Verification items for the finished model (mm, model axes). Face numbers are marked on the shaded views. A direction names the side the tool comes from. Give positions to 0.01 mm unless a question says otherwise; leave off trailing zeros. Loops run counter-clockwise (first coordinate to the right, second up) from the corner with the lowest first, then second, coordinate; pieces in that order, holes last. Notation, with made-up numbers: (-17, 9) - (1, 9) arc R8 ccw to (1, 14) - close; hole circle Ø9 at (6.5, 11). An arc over 180 degrees is marked (long way). One line per question, with ' | ' between items. Start each with the question number.
1. Tool access check on the marked faces 4, 5 and 6. Record the directions out of +Z, -Z, +X, -X, +Y, -Y that give a thin tool (end or side, any length) a straight path to the whole face; none if there is none.
2. Depth check by flat-ended pin: pin 1 Ø3 at (y, z) = (17.5, 1) entering from +X; pin 2 Ø1.5 at (y, z) = (29.5, 3.5) entering from -X; pin 3 Ø3 at (y, z) = (43, 4.5) entering from -X; pin 4 Ø3 at (y, z) = (24.5, 2) entering from +X. Enter the tip coordinate at first touch or a pass-through.
3. Section check B-B, the plane y = 9. Enter the section's corners in (x, z), then the cut area to 3 significant figures.
4. Thickness scan on line 1 along Y through (x, z) = (9.35, 3); line 2 along Z through (x, y) = (66.2, 25); line 3 along Y through (x, z) = (70, 0.75). Record the ranges inside material, lowest first. Write a range as from..to.
5. Section check A-A, the plane y = 25. Enter the section's corners in (x, z), then the cut area to 3 significant figures.
6. Mould release check, pull along Y, two halves, no side actions. Record for the marked faces 1, 2 and 3: +Y half, -Y half, draft (parallel to the pull), parting line (faces both ways), or undercut.
Autodesk Inventor part; units mm, degrees
ref_plane "YZ Plane" through (0, 0, 0) normal (1, 0, 0) x (0, 1, 0)
ref_plane "XZ Plane" through (0, 0, 0) normal (0, 1, 0) x (-1, 0, 0)
ref_plane "XY Plane" through (0, 0, 0) normal (0, 0, 1) x (1, 0, 0)
sketch "スケッチ1" plane through (0, 0, 0) normal (0, 0, 1) x (1, 0, 0)
  line L0 (0, 0) -> (75, 0)
  line L1 (75, 0) -> (75, 50)
  line L2 (75, 50) -> (0, 50)
  line L3 (0, 50) -> (0, 0)
  line L4 (0, 50) -> (7.5, 50)
  line L5 (7.5, 50) -> (7.5, 40)
  line L6 (7.5, 40) -> (0, 40)
  line L7 (0, 40) -> (0, 50)
  line L8 (75, 0) -> (0, 0)
  line L9 (0, 0) -> (0, 49.7722)
  line L10 (7.5, 0) -> (7.5, 10)
  line L11 (7.5, 10) -> (0, 10)
  line L12 (75, 0) -> (0, 0)
  line L13 (0, 50) -> (75, 50)
  line L14 (75, 50) -> (75, 0)
  line L15 (75, 50) -> (67.5, 50)
  line L16 (67.5, 50) -> (67.5, 40)
  line L17 (67.5, 40) -> (75, 40)
  line L18 (75, 40) -> (75, 50)
  line L19 (67.5, 0) -> (67.5, 10)
  line L20 (67.5, 10) -> (75, 10)
  line L21 (7.5, 30) -> (0, 30)
  line L22 (0, 30) -> (0, 20)
  line L23 (0, 20) -> (7.5, 20)
  line L24 (7.5, 20) -> (7.5, 30)
  line L25 (75, 50) -> (75, 0)
  line L26 (75, 0) -> (75, 49.7722)
  line L27 (67.5, 30) -> (75, 30)
  line L28 (75, 30) -> (75, 20)
  line L29 (75, 20) -> (67.5, 20)
  line L30 (67.5, 20) -> (67.5, 30)
  dimension "d0" = 75
  dimension "d1" = 50
  dimension "d2" = 7.5
  dimension "d3" = 10
  dimension "d4" = 10
  dimension "d5" = 10
extrude "押し出し1" add sketch "スケッチ1" along normal blind 6 contours L10 L11 L3 L23 L24 L21 L6 L5 L2 L16 L17 L1 L27 L30 L29 L20 L19 L0
sketch "スケッチ2" plane through (7.5, 20, 0) normal (-1, 0, 0) x (0, 0, 1)
  line L0 (0, 10) -> (6, 10)
  line L1 (0, 10) -> (0, 0)
  point P0 (0, -20)
  point P1 (3, 5)
  dimension "d8" = 5
  dimension "d9" = 3
sketch "スケッチ3" plane through (67.5, 20, 0) normal (1, 0, 0) x (0, 0, -1)
  line L0 (-6, 0) -> (-6, 10)
  line L1 (0, 10) -> (-6, 10)
  point P0 (0, -20)
  point P1 (-3, 5)
  dimension "d10" = 3
  dimension "d11" = 5
hole "穴1" at (67.5, 25, 3) direction (-1, 0, 0) diameter 4 depth 4.5
hole "穴2" at (7.5, 25, 3) direction (1, 0, 0) diameter 4 depth 4.5
fillet "フィレット1" radius 2 16 edges at (75, 35, 0) (75, 35, 6) (75, 40, 3) (75, 30, 3) (75, 20, 3) (75, 15, 6) (75, 15, 0) (75, 10, 3) (0, 35, 0) (0, 40, 3) (0, 35, 6) (0, 30, 3) (0, 20, 3) (0, 15, 0) (0, 10, 3) (0, 15, 6)
properties part number "menteA"
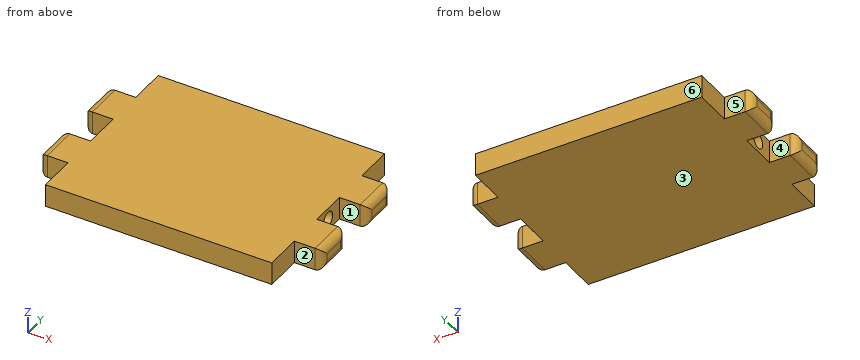
Results list:
1) face 4: +Z, -Z, -X | face 5: +Z, -Z, -X, +Y | face 6: +Z, -Z, +X, -X, +Y
2) pin 1: x = 75 | pin 2: x = 1.03 | pin 3: x = 7.5 | pin 4: x = 67.5
3) outline: (7.5, 0) - (67.5, 0) - (67.5, 6) - (7.5, 6) - close | area: 360 mm²
4) line 1: 0..23, 27..50 | line 2: 0..1, 5..6 | line 3: 10..20, 30..40
5) outline: (7.5, 0) - (67.5, 0) - (67.5, 1) - (63, 1) - (63, 5) - (67.5, 5) - (67.5, 6) - (7.5, 6) - (7.5, 5) - (12, 5) - (12, 1) - (7.5, 1) - close | area: 324 mm²
6) face 1: undercut | face 2: -Y half | face 3: draft
